Could you check a few things on this model? Use its own coordinates, in mm. A direction names the side the tool comes from. Give positions to 0.01 mm unless a question says otherwise; leave off trailing zeros.
(1) On a 3-axis mill with a long thin cutter (end or side, diameter ignored), from which of +Z, -Z, +X, -X, +Y, -Y can I reach the whole of each face in a straight line? I mean faces 1 (the flat face through (34, -22, -0.5)), 2 (the flat face through (37, -32, 0.125)), 3 (the flat face through (36, -27, -0.25)). Say none if no direction works.
(2) Will these pins go through, and if not, where does the flat tip stop? pin 1 (1 mm diameter, centred on x = 36, y = -32, fed in from -Z) (3 decimals); pin 2 (2 mm diameter, centred on x = 33.5, y = -29, fed in from +Z).
(3) If I drill on probe 1 along Z at (x, y) = (37.5, -30.5) (3 decimals); probe 2 along Y at (x, z) = (31.75, 0.3); probe 3 along Y at (x, z) = (35.5, 0.3), over which ranges is the centre line in solid material (lowest first)?
from build123d import *

# Parameters (mm, degrees)
F3_DEPTH = 0.5
F4_DEPTH = 0.25
F5_DEPTH = 0.125


with BuildPart() as f3:
    # F0 (on Top) → F3 (new body, symmetric)
    with BuildSketch(Plane.XY):
        with BuildLine():
            add(Edge.make_bspline(
                [(33.4646962583, -17.3531565815), (34.0183108685, -18.2014548185), (35.1449052053, -19.9277242701), (36.0757257814, -21.8882678628), (36.5491360426, -22.885389626)],
                knots=[0, 0, 0, 0, 0.4914054617, 1, 1, 1, 1], degree=3))
            Line((33.4646962583, -17.3531565815), (33.4646962583, -27.1025765687))
            add(Edge.make_bspline(
                [(36.5491360426, -22.885389626), (36.3445585773, -23.1038442345), (35.8796853463, -23.6002513022), (34.9096324661, -24.7869173938), (34.0141321874, -26.0750864021), (33.6374846111, -26.7794482037), (33.4646962583, -27.1025765687)],
                knots=[0, 0, 0, 0, 0.2146146816, 0.4876813793, 0.7649720955, 1, 1, 1, 1], degree=3))
        make_face()
        with BuildLine():
            Line((33.4646962583, -27.1025765687), (33.4646962583, -17.3531565815))
            add(Edge.make_bspline(
                [(33.4646962583, -17.3531565815), (32.9110816481, -18.2014548185), (31.7844873114, -19.9277242701), (30.8536667352, -21.8882678628), (30.380256474, -22.885389626)],
                knots=[0, 0, 0, 0, 0.4914054617, 1, 1, 1, 1], degree=3))
            add(Edge.make_bspline(
                [(30.380256474, -22.885389626), (30.5848339393, -23.1038442345), (31.0497071704, -23.6002513022), (32.0197600505, -24.7869173938), (32.9152603292, -26.0750864021), (33.2919079055, -26.7794482037), (33.4646962583, -27.1025765687)],
                knots=[0, 0, 0, 0, 0.2146146816, 0.4876813793, 0.7649720955, 1, 1, 1, 1], degree=3))
        make_face()
    extrude(amount=F3_DEPTH, both=True)

    # F1 (on Top) → F4 (join, symmetric)
    with BuildSketch(Plane.XY):
        with BuildLine():
            add(Edge.make_bspline(
                [(35.0542590022, -31.3443131745), (34.9321986711, -30.7857678371), (34.6969077554, -29.7078948129), (34.132815237, -28.3447046876), (33.7753301671, -27.5824159663), (33.5594348558, -27.2516943021), (33.4646962583, -27.1025765687)],
                knots=[0, 0, 0, 0, 0.3133220633, 0.6043357393, 0.8223308356, 1, 1, 1, 1], degree=3))
            add(Edge.make_bspline(
                [(35.0542590022, -31.3443131745), (35.2772294367, -30.9821031837), (35.7692332915, -30.1828550139), (37.0790252489, -28.6734392692), (37.7096471433, -28.1030367575), (37.986304611, -27.8527978808)],
                knots=[0, 0, 0, 0, 0.3174952829, 0.7005812383, 1, 1, 1, 1], degree=3))
            add(Edge.make_bspline(
                [(37.986304611, -27.8527978808), (37.8913761068, -27.3386059194), (37.6895959259, -26.2568236513), (37.1813869776, -24.4473320709), (36.7453139366, -23.3831491328), (36.5491360426, -22.885389626)],
                knots=[0, 0, 0, 0, 0.3227170226, 0.6711723471, 1, 1, 1, 1], degree=3))
            add(Edge.make_bspline(
                [(36.5491360426, -22.885389626), (36.3445585773, -23.1038442345), (35.8796853463, -23.6002513022), (34.9096324661, -24.7869173938), (34.0141321874, -26.0750864021), (33.6374846111, -26.7794482037), (33.4646962583, -27.1025765687)],
                knots=[0, 0, 0, 0, 0.2146146816, 0.4876813793, 0.7649720955, 1, 1, 1, 1], degree=3))
        make_face()
    extrude(amount=F4_DEPTH, both=True)

    # F2 (on Top) → F5 (join, symmetric)
    with BuildSketch(Plane.XY):
        with BuildLine():
            add(Edge.make_bspline(
                [(35.0099876523, -36.0890328884), (35.0691884535, -35.8017616591), (35.2086991521, -35.1286773781), (35.3078029344, -33.4406536261), (35.206077093, -32.2005833036), (35.0939553855, -31.6004826678), (35.0542590022, -31.3443131745)],
                knots=[0, 0, 0, 0, 0.2268047855, 0.5281413876, 0.7889814592, 1, 1, 1, 1], degree=3))
            add(Edge.make_bspline(
                [(35.0099876523, -36.0890328884), (35.1785122203, -35.7952578593), (35.5196858817, -35.1968595796), (36.1572480721, -34.2428839294), (36.8370476627, -33.5371282988), (37.5739759872, -32.8287365687), (37.8503923319, -32.5516161451), (37.986304611, -32.4345082045)],
                knots=[0, 0, 0, 0, 0.2099201912, 0.43002195, 0.637960627, 0.8451293142, 1, 1, 1, 1], degree=3))
            add(Edge.make_bspline(
                [(37.986304611, -32.4345082045), (38.0349117761, -32.091378108), (38.1858021608, -31.3817408763), (38.2103824602, -30.2099574058), (38.1870733454, -29.2358358547), (38.0405633584, -28.3246195438), (37.986304611, -27.8527978808)],
                knots=[0, 0, 0, 0, 0.2419441986, 0.4924070964, 0.724101854, 1, 1, 1, 1], degree=3))
            add(Edge.make_bspline(
                [(35.0542590022, -31.3443131745), (35.2772294367, -30.9821031837), (35.7692332915, -30.1828550139), (37.0790252489, -28.6734392692), (37.7096471433, -28.1030367575), (37.986304611, -27.8527978808)],
                knots=[0, 0, 0, 0, 0.3174952829, 0.7005812383, 1, 1, 1, 1], degree=3))
        make_face()
    extrude(amount=F5_DEPTH, both=True)


solid = f3.part
Answer block:
1. face 1: -Z, +X, -X, +Y, -Y
1. face 2: +Z, +X, -Y
1. face 3: -Z, +X, -Y
2. pin 1: stops at z = -0.125
2. pin 2: stops at z = 0.25
3. probe 1: z = -0.125 to 0.125
3. probe 2: y = -24.47 to -20.14
3. probe 3: y = -24.07 to -20.74
